Check sheet for the modelled part. Datum: model origin and axes. Units: mm. Round coordinates to 2 decimals unless told otherwise and drop trailing zeros. Loops run counter-clockwise (first coordinate to the right, second up) from the corner with the lowest first, then second, coordinate; pieces in that order, holes last. Notation, with made-up numbers: M 13,62 L 37,62 A14 ccw 37,76 Z; hole C -26,39 d6. An arc over 180 degrees is marked long. One line per question, with ' | ' between items. Start each with the question number.
(1) Section check B-B (z = 51). Record the boundary of the cut face in (x, y).
(2) Thickness scan on probe 1 along X at (y, z) = (26, -75); probe 2 along Z at (x, y) = (101.5, 23.5); probe 3 along X at (y, z) = (3.25, 117). Record the ranges inside material, lowest first. Write a range as [from, to].
(3) Go/stop test with flat-tipped pins: P1, Ø6, axis at y = 10.5, z = -37, coming from the +X side; P2, Ø10, axis at y = 9.5, z = 15, coming from the +X side; P3, Ø6, axis at x = -23, y = 11, coming from the +Z side. Record where each tip stops, or that it passes through.
(4) Section check C-C (y = 18). Count the separate pieces of the cut face and the enclosed holes in it, and give its area (3 significant figures).
(5) Section check A-A (x = 0). Record the boundary of the cut face in (y, z), and give its area (3 significant figures).
Autodesk Inventor part; units mm, degrees
ref_plane "YZ Plane" through (0, 0, 0) normal (1, 0, 0) x (0, 1, 0)
ref_plane "XZ Plane" through (0, 0, 0) normal (0, 1, 0) x (-1, 0, 0)
ref_plane "XY Plane" through (0, 0, 0) normal (0, 0, 1) x (1, 0, 0)
sketch "Sketch1" plane through (0, 0, 0) normal (0, 1, 0) x (-1, 0, 0)
  circle A0 centre (0, 0) radius 135
  circle A1 centre (0, 0) radius 110
  dimension "d0" = 270
  dimension "d1" = 220
extrude "Extrusion1" add sketch "Sketch1" along normal blind 30
sketch "Sketch2" plane through (0, 30, 0) normal (0, 1, 0) x (1, 0, 0)
  line L0 (-189, 0) -> (189, 0)
  point P0 (0, 0)
  point P1 (-125, 0)
  dimension "d11" = 125
hole "Hole1" at (-125, 30, 0) direction (0, -1, 0) diameter 5.2 end through all
pattern_circular "Circular Pattern1" count 10 over 360 about axis through (0, -10, 0) along (0, 1, 0) of "Hole1"
properties part number "Lower Ring (30mm)"
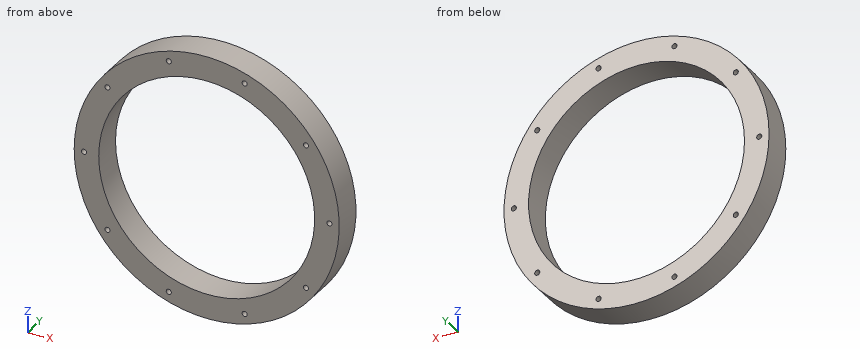
The answers:
1) outline: M -125,0 L -97.46,0 L -97.46,30 L -125,30 Z; M 97.46,0 L 125,0 L 125,30 L 97.46,30 Z
2) probe 1: [-112.25, -103.23], [-99.02, -80.47], [80.47, 99.02], [103.23, 112.25] | probe 2: [-89.01, -76.05], [-70.9, -42.4], [42.4, 70.9], [76.05, 89.01] | probe 3: [-67.35, -40.42], [-36.83, 36.83], [40.42, 67.35]
3) P1: x = 130.65 | P2: x = 134.63 | P3: z = 133.51
4) separate pieces: 1 | enclosed holes: 11 | area: 19,000 mm²
5) outline: M 0,-135 L 30,-135 L 30,-110 L 0,-110 Z; M 0,110 L 30,110 L 30,135 L 0,135 Z | area: 1,500 mm²
